from build123d import *

# Parameters (mm, degrees)
SKETCH1_R                  = 10
EXTRUDE_3_8_DEPTH          = 10
BOSS_EXTRUDE2_DEPTH        = 10
SKETCH3_R                  = 1.35
M3_DRILL_OR_THROUGH_DEPTH  = 10
FILLET1_R                  = 3
SKETCH4_R                  = 2.75
M5_THROUGH_DEPTH           = 8
SKETCH5_R                  = 2.2
M5_DRILL_DEPTH             = 8
CUT_EXTRUDE4_DEPTH         = 10
SKETCH7_R                  = 1.35
M3_DRILL_OR_THROUGH2_DEPTH = 10


with BuildPart() as part:
    # Sketch1 → 3/8 (new body)
    with BuildSketch(Plane.XY):
        with BuildLine():
            Line((-15, 0), (-15, 26.962387961))
            Line((-15, 26.962387961), (-23.034486956, 34.196672509))
            Line((-23.034486956, 34.196672509), (-17.681442105, 40.141831113))
            Line((-17.681442105, 40.141831113), (23.191523297, 3.339647763))
            Line((23.191523297, 3.339647763), (17.838478446, -2.605510841))
            Line((17.838478446, -2.605510841), (11.147172382, -10.036959095))
            ThreePointArc((11.147172382, -10.036959095), (-5.375519243, -14.003706397), (-15, 0))
        make_face()
        Circle(SKETCH1_R, mode=Mode.SUBTRACT)
    extrude(amount=EXTRUDE_3_8_DEPTH)

    # Sketch2 → Boss-Extrude2 (add)
    with BuildSketch(Plane.XY):
        Polygon((-8.703298337, -12.216898054), (-1.18575737, -14.953059201), (-5.28999909, -26.22937065), (-12.807540057, -23.493209503), align=None)
    extrude(amount=BOSS_EXTRUDE2_DEPTH)

    # Sketch3 → M3_DRILL_or_Through (cut)
    with BuildSketch(Plane.XY.offset(10)):
        with Locations((-7.524443153, -20.673237657)):
            Circle(SKETCH3_R)
    extrude(amount=-M3_DRILL_OR_THROUGH_DEPTH, mode=Mode.SUBTRACT)

    # Fillet1
    fillet1_edges = [part.edges().sort_by_distance(p)[0] for p in [
        (-12.807540057, -23.493209503, 5),
        (-5.28999909, -26.22937065, 5),
    ]]
    fillet(fillet1_edges, radius=FILLET1_R)

    # Sketch4 → M5_through (cut)
    with BuildSketch(Plane(origin=(12.044350914, 13.376606859, 0), x_dir=(0.7431448254773932, -0.6691306063588595, 0), z_dir=(0.6691306063588595, 0.7431448254773932, 0))):
        with Locations(Location((-35, -5, 0), (0, 0, 180))):
            Circle(SKETCH4_R)
    extrude(amount=-M5_THROUGH_DEPTH, mode=Mode.SUBTRACT)

    # Sketch5 → M5_DRILL (cut)
    with BuildSketch(Plane(origin=(12.044350914, 13.376606859, 0), x_dir=(0.7431448254773932, -0.6691306063588595, 0), z_dir=(0.6691306063588595, 0.7431448254773932, 0))):
        with Locations(Location((-15, -5, 0), (0, 0, 180))):
            Circle(SKETCH5_R)
        with Locations(Location((10, -5, 0), (0, 0, 180))):
            Circle(SKETCH5_R)
    extrude(amount=-M5_DRILL_DEPTH, mode=Mode.SUBTRACT)

    # Sketch6 → Cut-Extrude4 (cut)
    with BuildSketch(Plane.XY.offset(10)):
        with BuildLine():
            Line((-11, 20.669506324), (-11, 8.660254038))
            ThreePointArc((-11, 8.660254038), (-7.515689996, 11.81162156), (-3.18503916, 13.632883978))
            Line((-3.18503916, 13.632883978), (-11, 20.669506324))
        make_face()
    extrude(amount=-CUT_EXTRUDE4_DEPTH, mode=Mode.SUBTRACT)

    # Sketch7 → M3_DRILL_or_Through2 (cut)
    with BuildSketch(Plane.XY.offset(10)):
        with Locations((-7.654346968, 24.385230452)):
            Circle(SKETCH7_R)
    extrude(amount=-M3_DRILL_OR_THROUGH2_DEPTH, mode=Mode.SUBTRACT)


solid = part.part
Can you work these out from the model? Positions are in its coordinate system, mm. A direction names the side the tool comes from. Coordinates: 2 decimals unless noted, no trailing zeros. Loops run counter-clockwise (first coordinate to the right, second up) from the corner with the lowest first, then second, coordinate; pieces in that order, holes last. Notation, with made-up numbers: M 57,33.5 L 99,33.5 A29 cw 99,63.5 Z; hole C -13,-11.5 d7. An arc over 180 degrees is marked long. Return JSON: item names as keys, results as strings. Group by question number.
Item 1: On a 3-axis mill with a long thin cutter (end or side, diameter ignored), from which of +Z, -Z, +X, -X, +Y, -Y can I reach the whole of each face in a straight line? I mean faces 5 (the flat face through (-11, 15, 5)), 6 (the flat face through (-15, 13, 5)), 7 (the cylindrical face through (-5.85, -25.12, 5.07)). Say none if no direction works.
Item 2: Thinking about a two-plate mould opening in Z: for faces 1 (the flat face through (-2, 10, 0)), 2 (the cylindrical face through (18.04, 2.67, 6.49)), 3 (the cylindrical face through (-13.287, -6.961, 4.93)), 4 (the cylindrical face through (-16.162, 33.466, 2.315)), which applies, released by +Z, released by -Z, zero draft, split by the parting line, or undercut?
Item 3: Imagine slicing it at A-A (z = 3.75). Give the number of separate pieces and of enclosed holes in the cut face, and give its area (3 significant figures).
Item 4: I'm going to push flat-ended pins straight in: pin 1 Ø1.5 at (y, z) = (-13.5, 1) entering from +X; pin 2 Ø3 at (x, z) = (-3, 6) entering from +Y; pin 3 Ø6 at (x, z) = (-0.5, 3) entering from +Y; pin 4 Ø1.6 at (x, y) = (-7.52, -20.67) entering from -Z (3 decimals). Where does each tip first touch, or does it pass through?
Item 5: If I drill on L1, parallel to X at y = 34, z = 3; L2, parallel to X at y = 11, z = 9.5; L3, parallel to Y at x = 2, z = 8.75, over which ranges is the centre line in solid material (lowest first)? Write a range as from..to.
Item 6: Imagine slicing it at B-B (x = 9). Please give me the cut outline in (y, z).
Verdict:
{
 "1": {"face 5": "+Z, -Z", "face 6": "+Z, -Z, -X, -Y", "face 7": "+Z, -Z, -Y"},
 "2": {"face 1": "released by -Z", "face 2": "undercut", "face 3": "zero draft", "face 4": "undercut"},
 "3": {"separate pieces": "2", "enclosed holes": "4", "area": "834 mm^2"},
 "4": {"pin 1": "stops at x = 7.9", "pin 2": "stops at y = 28.27", "pin 3": "stops at y = 27.37", "pin 4": "passes through"},
 "5": {"L1": "x = -22.82..-19.02, -13.94..-10.86", "L2": "x = -15..-11, -8.66..14.68", "L3": "y = -14.87..-9.8, 9.8..22.42"},
 "6": {"outline": "M -12,0 L -4.36,0 L -4.36,10 L -12,10 Z; M 4.36,0 L 16.12,0 L 16.12,10 L 4.36,10 Z"}
}
